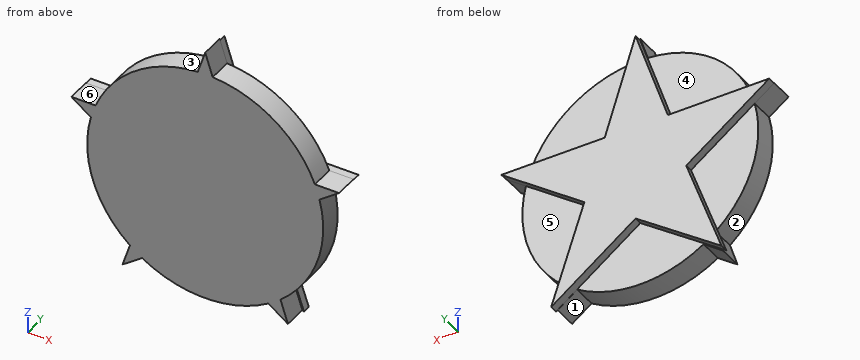
```python
from build123d import *

# Parameters (mm, degrees)
F0_R     = 38.1
F1_DEPTH = 7.62
F3_DEPTH = 7.62
F5_DEPTH = 2.54


with BuildPart() as f1:
    # F0 (on Front) → F1 (new body)
    with BuildSketch(Plane.XZ):
        Circle(F0_R)
    extrude(amount=F1_DEPTH)

    # F2 (on Front) → F3 (join)
    with BuildSketch(Plane.XZ):
        Polygon((43.2237411543, 14.0442448459), (10.2037411543, 14.0442448459), (16.51, -5.3644241848), align=None)
        Polygon((16.51, -5.3644241848), (10.2037411543, 14.0442448459), (-10.2037411543, 14.0442448459), (-16.51, -5.3644241848), (0, -17.3596413222), align=None)
        Polygon((-10.2037411543, 14.0442448459), (10.2037411543, 14.0442448459), (0, 45.448131014), align=None)
        Polygon((26.7137411543, -36.7683103529), (16.51, -5.3644241848), (0, -17.3596413222), align=None)
        Polygon((-16.51, -5.3644241848), (-10.2037411543, 14.0442448459), (-43.2237411543, 14.0442448459), align=None)
        Polygon((-26.7137411543, -36.7683103529), (0, -17.3596413222), (-16.51, -5.3644241848), align=None)
    extrude(amount=F3_DEPTH)

    # F4 (on face) → F5 (join)
    with BuildSketch(Plane.XZ):
        Polygon((16.5334772319, -5.4629510269), (9.9479760975, 13.9897912741), (-10.4440292343, 13.9897912741), (-16.3596607745, -5.4629510269), (0, -17.2653142363), align=None)
        Polygon((43.3266088367, 13.9897912741), (9.9479760975, 13.9897912741), (16.5334772319, -5.4629510269), align=None)
        Polygon((-10.4440292343, 13.9897912741), (9.9479760975, 13.9897912741), (0, 44.8327288032), align=None)
        Polygon((-16.3596607745, -5.4629510269), (-10.4440292343, 13.9897912741), (-43.1872978806, 13.9897912741), align=None)
        Polygon((27.2381013996, -37.0830648364), (16.5334772319, -5.4629510269), (0, -17.2653142363), align=None)
        Polygon((0, -17.2653142363), (-16.3596607745, -5.4629510269), (-27.761925516, -37.0830648364), align=None)
    extrude(amount=-F5_DEPTH)


solid = f1.part
```
Geometry: final body of the model. Coordinates: model frame, mm. Face numbers are marked on the shaded views. A direction names the side the tool comes from. Coordinates: 2 decimals unless noted, no trailing zeros. Loops run counter-clockwise (first coordinate to the right, second up) from the corner with the lowest first, then second, coordinate; pieces in that order, holes last. Notation, with made-up numbers: (16, -32) -> (26, -32) arc R25 ccw to (26, 7) -> close; hole circle Ø4 at (15.5, 60). An arc over 180 degrees is marked (long way). Use a Markdown table: item, result. Add a question column.
(1) Mould query, pull axis Z, two halves, no side actions, for the marked faces 1, 2 and 3. Classes: pulls with the +Z half, pulls with the -Z half, needs draft (parallel to the pull), parting line crosses it, or undercut.
(2) Section query C-C, the plane x = 19. Return loops of the section in (y, z).
(3) Section query D-D, the plane z = 37. Return loops of the section in (x, y), plus the area to 3 significant figures.
(4) Section query B-B, the plane z = -23. Return loops of the section in (x, y), plus the area to 3 significant figures.
(5) Section query A-A, the plane y = -1.5. Return loops of the section in (x, z), plus the area to 3 significant figures.
(6) Line query: line 1 along Z through (x, y) = (13, 2.25); line 2 along X through (y, z) = (-3.5, -34.5); line 3 along Y through (x, z) = (-23, 28). Output: solid intervals per line, ascending.
(7) Pin query (flat end, axial travel): pin 1 Ø5 at (y, z) = (-4, -14.5) entering from -X; pin 2 Ø1 at (y, z) = (-2.5, -22.5) entering from -X; pin 3 Ø6.5 at (x, z) = (10.5, -32.5) entering from +Y; pin 4 Ø1.5 at (x, z) = (26.5, -31) entering from -Y. Return the tip coordinate at first contact, or that it passes through.
(8) Access query for the marked faces 4, 5 and 6. Directions: +Z, -Z, +X, -X, +Y, -Y. A direction counts if a zero-diameter tool reaches every point of the face in a straight line with its end or side. Return the directions, or none.
Answer:
| question | item | result |
|---|---|---|
| 1 | face 1 | pulls with the -Z half |
| 1 | face 2 | undercut |
| 1 | face 3 | pulls with the +Z half |
| 2 | outline | (-7.62, -33.02) -> (0, -33.02) -> (0, -31.09) -> (2.54, -31.09) -> (2.54, -12.75) -> (0, -12.75) -> (0, -3.67) -> (2.54, -3.67) -> (2.54, 13.99) -> (0, 13.99) -> (0, 33.02) -> (-7.62, 33.02) -> close |
| 3 | outline | (-9.09, -7.62) -> (9.09, -7.62) -> (9.09, 0) -> (2.53, 0) -> (2.53, 2.54) -> (-2.65, 2.54) -> (-2.65, 0) -> (-9.09, 0) -> close |
| 3 | area | 152 mm^2 |
| 4 | outline | (-30.37, -7.62) -> (30.37, -7.62) -> (30.37, 0) -> (22.47, 0) -> (22.47, 2.54) -> (7.88, 2.54) -> (7.88, 0) -> (-8.03, 0) -> (-8.03, 2.54) -> (-22.68, 2.54) -> (-22.68, 0) -> (-30.37, 0) -> close |
| 4 | area | 537 mm^2 |
| 5 | outline | (-43.22, 14.04) -> (-36.91, 9.46) arc R38.1 ccw to (-24.3, -29.34) -> (-26.71, -36.77) -> (-20.4, -32.18) arc R38.1 ccw to (20.4, -32.18) -> (26.71, -36.77) -> (24.3, -29.34) arc R38.1 ccw to (36.91, 9.46) -> (43.22, 14.04) -> (35.42, 14.04) arc R38.1 ccw to (2.41, 38.02) -> (0, 45.45) -> (-2.41, 38.02) arc R38.1 ccw to (-35.42, 14.04) -> close |
| 5 | area | 4,650 mm^2 |
| 6 | line 1 | z = -26.72 to 13.99 |
| 6 | line 2 | x = -25.98 to -23.59, -16.17 to 16.17, 23.59 to 25.98 |
| 6 | line 3 | y = -7.62 to 0 |
| 7 | pin 1 | stops at x = -36.16 |
| 7 | pin 2 | stops at x = -31.11 |
| 7 | pin 3 | stops at y = 0 |
| 7 | pin 4 | passes through |
| 8 | face 4 | +Z, +Y |
| 8 | face 5 | +X, +Y |
| 8 | face 6 | +Z, -X, +Y, -Y |
